Autodesk Fusion 360 part; units mm, degrees
sketch "Skizze1" plane through (0, 0, 0) normal (0, 1, 0) x (1, 0, 0)
  arc A0 (0, 2) -> (2, 0) centre (2, 2) ccw
  arc A1 (2, 23) -> (0, 21) centre (2, 21) ccw
  line L0 (58.5, 23) -> (2, 23)
  line L1 (60.5, 2) -> (60.5, 21)
  arc A2 (58.5, 0) -> (60.5, 2) centre (58.5, 2) ccw
  line L2 (2, 0) -> (58.5, 0)
  line L3 (0, 21) -> (0, 2)
  arc A3 (60.5, 21) -> (58.5, 23) centre (58.5, 21) ccw
  point P0 (60.5, 0)
  point P1 (0, 23)
  dimension "d1" = 60.5
  dimension "d2" = 23
  dimension "d3" = 2
  dimension "d4" = 2
  dimension "d5" = 2
  dimension "d6" = 2
sketch "Skizze2" plane through (0, 0, 0) normal (0, 1, 0) x (1, 0, 0)
  line L0 (2.5, 1.5) -> (58, 1.5)
  line L1 (59, 2.5) -> (59, 20)
  line L2 (58, 21) -> (2.5, 21)
  line L3 (1.5, 20) -> (1.5, 2.5)
  line L4 (2, 0) -> (58.5, 0)
  line L5 (0, 21) -> (0, 2)
  arc A0 (2.5, 21) -> (1.5, 20) centre (2.5, 20) ccw
  arc A1 (1.5, 2.5) -> (2.5, 1.5) centre (2.5, 2.5) ccw
  arc A2 (59, 20) -> (58, 21) centre (58, 20) ccw
  arc A3 (58, 1.5) -> (59, 2.5) centre (58, 2.5) ccw
  point P0 (1.5, 1.5)
  point P1 (59, 1.5)
  point P2 (1.5, 21)
  dimension "d7" = 57.5
  dimension "d8" = 19.5
  dimension "d9" = 1.5
  dimension "d10" = 1.5
  dimension "d11" = 1
sketch "Skizze3" plane through (0, 0, 0) normal (0, 1, 0) x (1, 0, 0)
  line L0 (24, 17) -> (24, 5.8)
  line L1 (36.5, 17) -> (24, 17)
  line L2 (36.5, 5.8) -> (36.5, 17)
  line L3 (24, 5.8) -> (36.5, 5.8)
  line L4 (0, 21) -> (0, 2)
  line L5 (2, 0) -> (58.5, 0)
  dimension "d12" = 12.5
  dimension "d13" = 11.2
  dimension "d14" = 24
  dimension "d15" = 5.8
sketch "Skizze4" plane through (0, 0, 0) normal (0, 1, 0) x (1, 0, 0)
  circle A0 centre (44.5, 11.6) radius 1.425
  circle A1 centre (49.5, 11.6) radius 1.425
  circle A2 centre (54.5, 11.6) radius 1.425
  line L0 (2.5, 1.5) -> (58, 1.5)
  line L1 (24, 17) -> (24, 5.8)
  line L2 (36.5, 5.8) -> (36.5, 17)
  line L3 (2, 0) -> (58.5, 0)
  dimension "d16" = 2.85
  dimension "d17" = 2.85
  dimension "d18" = 2.85
  dimension "d19" = 5
  dimension "d20" = 5
  dimension "d25" = 8
  dimension "d26" = 11.6
extrude "Extrusion1" add sketch "Skizze1" along normal blind 1.6
extrude "Extrusion2" add sketch "Skizze2" along normal blind 2.6
extrude "Extrusion3" cut sketch "Skizze4" sketch "Skizze3" along normal blind 2.6 of sketch 2
equation "h1 = 3 mm"
equation "h1_hoehe = 6.5 mm"
The model under review builds one solid part; all positions refer to its coordinate system, in mm. A direction names the side the tool comes from. Round coordinates to 2 decimals unless told otherwise and drop trailing zeros. Write each loop counter-clockwise with the first axis right and the second up, starting at its lowest first coordinate (ties: lowest second). Pieces come first, ordered by that corner, then holes. Notation, with made-up numbers: M 49.5,47 L 86.5,47 A16 cw 86.5,69 Z; hole C 16,49.25 d6. An arc over 180 degrees is marked long. Use a Markdown table: item, result. Add a question column.
Q1. Insertion check: pin 1 (1.3 mm diameter, centred on y = 1, z = -10, fed in from -X); pin 2 (0.5 mm diameter, centred on y = 2, z = -10.5, fed in from +X). Each pin has a flat end and moves straight along its axis. Give the tip position at first contact, or say it passes through.
Q2. The part is to be moulded in two halves that separate along Z. For faces 1 (the face through (59.93, 0.79, -0.6)), 2 (the face through (53.076, 1.282, -11.537)), 3 (the face through (59.9, 0.79, -22.43)), say which applies: pulls with the +Z half, pulls with the -Z half, needs draft (parallel to the pull), parting line crosses it, or undercut.
Q3. To check wall thickness, follow line 1 (X direction, y = 1.15, z = -11.6) (3 decimals); line 2 (X direction, y = 1.9, z = -11.6) (3 decimals); line 3 (Z direction, x = 54.5, y = 1.1) (3 decimals). State the ranges of each line that lie inside material, in increasing order.
Q4. We need section D-D, the plane y = 0.5. State the section outline as (x, z) points (3 decimals), plus the area to 3 significant figures.
Q5. We need section B-B, the plane z = -11.6. State the section outline as (x, y) points (3 decimals), plus the area to 3 significant figures.
Q6. Machinability: for faces 4 (the face through (31, 2, -21)), 5 (the face through (1.801, 2.093, -1.785)), 6 (the face through (36.5, 1, -11)), 7 (the face through (30, 2, -1.5)), 8 (the face through (58.715, 2.093, -1.801)), which of the approach directions +Z, -Z, +X, -X, +Y, -Y give a long, thin tool a straight path to every point of the face, cutting with its end or side? Answer none if there is none.
Q7. We need section A-A, the plane x = 35. State the section outline as (y, z) points, plus the area to 3 significant figures.
Q8. We need section C-C, the plane z = -14. State the section outline as (x, y) points.
Findings below:
| question | item | result |
|---|---|---|
| 1 | pin 1 | stops at x = 0 |
| 1 | pin 2 | stops at x = 59 |
| 2 | face 1 | pulls with the +Z half |
| 2 | face 2 | undercut |
| 2 | face 3 | pulls with the -Z half |
| 3 | line 1 | x = 0 to 24, 36.5 to 43.075, 45.925 to 48.075, 50.925 to 53.075, 55.925 to 60.5 |
| 3 | line 2 | x = 1.5 to 24, 36.5 to 43.075, 45.925 to 48.075, 50.925 to 53.075, 55.925 to 59 |
| 3 | line 3 | z = -23 to -13.025, -10.175 to 0 |
| 4 | outline | M 0,-21 A2 ccw 2,-23 L 58.5,-23 A2 ccw 60.5,-21 L 60.5,-2 A2 ccw 58.5,0 L 2,0 A2 ccw 0,-2 Z; hole M 24,-17 L 36.5,-17 L 36.5,-5.8 L 24,-5.8 Z; hole C 44.5,-11.6 d2.85; hole C 49.5,-11.6 d2.85; hole C 54.5,-11.6 d2.85 |
| 4 | area | 1,230 mm² |
| 5 | outline | M 0,0 L 24,0 L 24,2.6 L 1.5,2.6 L 1.5,1.6 L 0,1.6 Z; M 36.5,0 L 43.075,0 L 43.075,2.6 L 36.5,2.6 Z; M 45.925,0 L 48.075,0 L 48.075,2.6 L 45.925,2.6 Z; M 50.925,0 L 53.075,0 L 53.075,2.6 L 50.925,2.6 Z; M 55.925,0 L 60.5,0 L 60.5,1.6 L 59,1.6 L 59,2.6 L 55.925,2.6 Z |
| 5 | area | 99.6 mm² |
| 6 | face 4 | -Z, +X, -X, +Y |
| 6 | face 5 | +Z, -X, +Y |
| 6 | face 6 | +Y, -Y |
| 6 | face 7 | +Z, +X, -X, +Y |
| 6 | face 8 | +Z, +X, +Y |
| 7 | outline | M 0,-23 L 1.6,-23 L 1.6,-21 L 2.6,-21 L 2.6,-17 L 0,-17 Z; M 0,-5.8 L 2.6,-5.8 L 2.6,-1.5 L 1.6,-1.5 L 1.6,0 L 0,0 Z |
| 7 | area | 27.2 mm² |
| 8 | outline | M 0,0 L 24,0 L 24,2.6 L 1.5,2.6 L 1.5,1.6 L 0,1.6 Z; M 36.5,0 L 60.5,0 L 60.5,1.6 L 59,1.6 L 59,2.6 L 36.5,2.6 Z |
